Here's how the part is built. I have some questions about the finished solid (model axes, mm). A direction names the side the tool comes from. Give positions to 0.01 mm unless a question says otherwise; leave off trailing zeros. Order: outer loops, then holes, each group sorted by start corner. A loop starts at its lowest first (then second) coordinate and runs counter-clockwise, first axis right, second up. Notation, with made-up numbers: (11.25, -29.75) -> (66.25, -29.75) arc R29 ccw to (66.25, -5.75) -> close; hole circle Ø1 at (37, -12.75). An arc over 180 degrees is marked (long way). Write each question's results on one line, items separated by ' | '. Start each with the question number.
Q1. Imagine slicing it at B-B, the plane y = 16.5. Please give me the cut outline in (x, z), then the cut area to 3 significant figures.
Q2. For faces 5 (the face through (-3, 7, 4)), 6 (the face through (17.292, -1.352, 3.303)), 7 (the face through (0.17, 4.5, 9.2)), which set-ups out of +Z, -Z, +X, -X, +Y, -Y let a thin tool reach every point of the face, with its end or its side?
Q3. Imagine slicing it at D-D, the plane x = 0. Please give me the cut outline in (y, z), then the cut area to 3 significant figures.
Q4. Thinking about a two-plate mould opening in X: for faces 1 (the face through (10.07, 28.1, 0.99)), 2 (the face through (0.1, 0, 11.2)), 3 (the face through (0, 41, 1)), 4 (the face through (0, -2.95, 11)), which applies, pulls with the +X half, pulls with the -X half, needs draft (parallel to the pull), parting line crosses it, or undercut?
Q5. Imagine slicing it at C-C, the plane y = 0. State how many separate pieces and enclosed holes the cut face has, then the cut area to 3 significant figures.
Q6. I need wall thicknesses on line 1 along Y through (x, z) = (13, 9.25); line 2 along X through (y, z) = (0, 14.75); line 3 along Z through (x, y) = (24.5, -13.5). Which ranges of each line are inside material? Lowest first, please. Write a range as [from, to].
Q7. I'm going to push flat-ended pins straight in: pin 1 (5 mm diameter, centred on x = 2, y = -11, fed in from +Z); pin 2 (2 mm diameter, centred on x = 15, z = 1, fed in from +Y); pin 3 (8.5 mm diameter, centred on x = 3, z = 13, fed in from -Y). Where does each tip first touch, or does it pass through?
```python
from build123d import *

# Parameters (mm, degrees)
F0_W          = 38
F0_H          = 12
F0_R          = 2.2
F1_DEPTH      = 16.8
F3_DEPTH      = 12.001
F4_R          = 8.1
F5_DEPTH      = 3.05
F6_R          = 8.1
F7_DEPTH      = 3.05
F8_R          = 16.345
F9_DEPTH      = 2
F10_R         = 1.45
F11_DEPTH     = 16.801
F12_R         = 4.5
F12_R_2       = 2.2
F13_DEPTH     = 9
F14_SIZE      = 2.29999
F15_T4_DEPTH  = 23.6674466009
F15_S5_R      = 16.345
F15_T6_DEPTH  = 14
F15_S7_R      = 1.45
F15_T8_DEPTH  = 14
F15_T12_DEPTH = 38.54569481
F15_S13_R     = 25
F15_T14_DEPTH = 21
F15_S15_R     = 16.345
F15_T16_DEPTH = 21
F16_T1_DEPTH  = 2
F16_T3_DEPTH  = 26.8


# Not quite as in the source:
# - a fillet or chamfer that OpenCascade refuses, or shapes differently, is made with other operations: its cross-section is extruded or revolved along the edge and cut away or added
# - a fillet or chamfer is up to 0.001 mm smaller than in the source, because OpenCascade refuses the exact size


with BuildPart() as f1:
    # F0 (on Top) → F1 (new body)
    with BuildSketch(Plane.XY):
        Rectangle(F0_W, F0_H)
        with Locations((-13, 0)):
            Circle(F0_R, mode=Mode.SUBTRACT)
        with Locations((13, 0)):
            Circle(F0_R, mode=Mode.SUBTRACT)
    extrude(amount=F1_DEPTH)

    # F2 (on face) → F3 (cut, through all)
    with BuildSketch(Plane(origin=(0, 6, 0), x_dir=(-1, 0, 0), z_dir=(0, 1, 0))):
        with BuildLine():
            ThreePointArc((-6.0794736614, 16.8), (0, 11.2), (6.0794736614, 16.8))
            Line((6.0794736614, 16.8), (-6.0794736614, 16.8))
        make_face()
        with BuildLine():
            Line((-6.0794736614, 16.8), (6.0794736614, 16.8))
            ThreePointArc((6.0794736614, 16.8), (6.0948662551, 17.0497894234), (6.1, 17.3))
            ThreePointArc((6.1, 17.3), (-0.2502105766, 23.3948662551), (-6.0794736614, 16.8))
        make_face()
    extrude(amount=-F3_DEPTH, mode=Mode.SUBTRACT)

    # F4 (on face) → F5 (cut)
    with BuildSketch(Plane(origin=(0, 6, 0), x_dir=(-1, 0, 0), z_dir=(0, 1, 0))):
        with Locations((0, 17.3)):
            Circle(F4_R)
    extrude(amount=-F5_DEPTH, mode=Mode.SUBTRACT)

    # F6 (on face) → F7 (cut)
    with BuildSketch(Plane.XZ.offset(6)):
        with Locations((0, 17.3)):
            Circle(F6_R)
    extrude(amount=-F7_DEPTH, mode=Mode.SUBTRACT)

    # F8 (on Top) → F9 (join)
    with BuildSketch(Plane.XY):
        with BuildLine():
            Line((-9.5, 41), (-9.5, 4))
            ThreePointArc((-9.5, 4), (29.848439809, -16.4722441189), (24.03, 27.5))
            Line((24.03, 27.5), (9.5, 27.5))
            Line((9.5, 27.5), (9.5, 41))
            Line((9.5, 41), (-9.5, 41))
        make_face()
        with Locations((17.995, 5.245)):
            Circle(F8_R, mode=Mode.SUBTRACT)
    extrude(amount=F9_DEPTH)

    # F10 (on face) → F11 (cut, through all)
    with BuildSketch(Plane(origin=(0, 0, 0), x_dir=(1, 0, 0), z_dir=(0, 0, -1))):
        with Locations((-5, -10.5)):
            Circle(F10_R)
        with Locations((-5, -25.5)):
            Circle(F10_R)
    extrude(amount=-F11_DEPTH, mode=Mode.SUBTRACT)

    # F12 (on face) → F13 (cut)
    with BuildSketch(Plane(origin=(0, 0, 0), x_dir=(1, 0, 0), z_dir=(0, 0, -1))):
        with Locations((-13, 0)):
            Circle(F12_R)
        with Locations((-13, 0)):
            Circle(F12_R_2, mode=Mode.SUBTRACT)
        with Locations((13, 0)):
            Circle(F12_R)
        with Locations((13, 0)):
            Circle(F12_R_2, mode=Mode.SUBTRACT)
    extrude(amount=-F13_DEPTH, mode=Mode.SUBTRACT)

    # F14 (size 2.3 in the source; OpenCascade refuses exactly that, so slightly less here)
    f14_edges = [f1.edges().sort_by_distance(p)[0] for p in [
        (-17.5, 0, 9),
        (8.5, 0, 9),
    ]]
    chamfer(f14_edges, length=F14_SIZE)

    # F15: fillet of radius 5 on 2 edges, made by hand


with BuildPart() as f15_tool2:
    # F15_s3 → F15_t4 (new body)
    with BuildSketch(Plane.YZ.offset(14.1674466009)):
        with BuildLine():
            ThreePointArc((6, 7), (7.4644660941, 3.4644660941), (11, 2))
            Line((11, 2), (6, 2))
            Line((6, 2), (6, 7))
        make_face()
    extrude(amount=-F15_T4_DEPTH)

    # F15_s5 → F15_t6 (cut, symmetric)
    with BuildSketch(Plane.XY.offset(4.5)):
        with Locations((17.995, 5.245)):
            Circle(F15_S5_R)
    extrude(amount=F15_T6_DEPTH, both=True, mode=Mode.SUBTRACT)

    # F15_s7 → F15_t8 (cut, symmetric)
    with BuildSketch(Plane.XY.offset(4.5)):
        with Locations((-5, 10.5)):
            Circle(F15_S7_R)
    extrude(amount=F15_T8_DEPTH, both=True, mode=Mode.SUBTRACT)


with BuildPart() as f1_1:
    add(f1.part)

    # F15_t1: union F15_tool2
    add(f15_tool2.part)


with BuildPart() as f15_tool10:
    # F15_s11 → F15_t12 (new body)
    with BuildSketch(Plane.YZ.offset(-19.9127772578)):
        with BuildLine():
            ThreePointArc((-6, 7), (-7.4644660941, 3.4644660941), (-11, 2))
            Line((-11, 2), (-6, 2))
            Line((-6, 2), (-6, 7))
        make_face()
    extrude(amount=F15_T12_DEPTH)

    # F15_s13 → F15_t14 (intersect, symmetric)
    with BuildSketch(Plane.XY.offset(4.5)):
        with Locations((15.4999999989, 4.0002319164)):
            Circle(F15_S13_R)
    extrude(amount=F15_T14_DEPTH, both=True, mode=Mode.INTERSECT)

    # F15_s15 → F15_t16 (cut, symmetric)
    with BuildSketch(Plane.XY.offset(4.5)):
        with Locations((17.995, 5.245)):
            Circle(F15_S15_R)
    extrude(amount=F15_T16_DEPTH, both=True, mode=Mode.SUBTRACT)


with BuildPart() as f1_2:
    add(f1_1.part)

    # F15_t9: union F15_tool10
    add(f15_tool10.part)

    # F16: fillet of radius 2 on 5 edges, made by hand

    # F16_s2 → F16_t1 (join)
    with BuildSketch(Plane.XY):
        with BuildLine():
            ThreePointArc((9.5, 29.5), (10.0857864376, 28.0857864376), (11.5, 27.5))
            Line((11.5, 27.5), (9.5, 27.5))
            Line((9.5, 27.5), (9.5, 29.5))
        make_face()
    extrude(amount=F16_T1_DEPTH)

    # F16_s4 → F16_t3 (cut)
    with BuildSketch(Plane.XY.offset(-5)):
        with BuildLine():
            ThreePointArc((17, 6), (18.4142135624, 5.4142135624), (19, 4))
            Line((19, 4), (19, 6))
            Line((19, 6), (17, 6))
        make_face()
        with BuildLine():
            ThreePointArc((17, -6), (18.4142135624, -5.4142135624), (19, -4))
            Line((19, -4), (19, -6))
            Line((19, -6), (17, -6))
        make_face()
        with BuildLine():
            ThreePointArc((-19, 4), (-18.4142135624, 5.4142135624), (-17, 6))
            Line((-17, 6), (-19, 6))
            Line((-19, 6), (-19, 4))
        make_face()
        with BuildLine():
            ThreePointArc((-17, -6), (-18.4142135624, -5.4142135624), (-19, -4))
            Line((-19, -4), (-19, -6))
            Line((-19, -6), (-17, -6))
        make_face()
    extrude(amount=F16_T3_DEPTH, mode=Mode.SUBTRACT)


solid = f1_2.part
```
Geometry check:
1) outline: (-9.5, 0) -> (6.14, 0) -> (6.14, 2) -> (-9.5, 2) -> close; (29.85, 0) -> (37.15, 0) -> (37.15, 2) -> (29.85, 2) -> close | area: 45.9 mm²
2) face 5: +Z, +X, -X, +Y | face 6: -Z | face 7: +Z, +Y
3) outline: (-15.61, 0) -> (41, 0) -> (41, 2) -> (11, 2) arc R5 cw to (6, 7) -> (6, 9.2) -> (2.95, 9.2) -> (2.95, 11.2) -> (-2.95, 11.2) -> (-2.95, 9.2) -> (-6, 9.2) -> (-6, 7) arc R5 cw to (-11, 2) -> (-15.61, 2) -> close | area: 222 mm²
4) face 1: pulls with the +X half | face 2: undercut | face 3: needs draft | face 4: undercut
5) separate pieces: 4 | enclosed holes: 0 | area: 379 mm²
6) line 1: [-6, -2.2], [2.2, 6] | line 2: [-19, -15.2], [-10.8, -5.54], [5.54, 10.8], [15.2, 19] | line 3: [0, 2]
7) pin 1: z = 2.67 | pin 2: y = 27.5 | pin 3: y = -6
